The listing builds one solid part. Answer for the finished solid, in the listing's coordinates (mm). Face numbers are marked on the shaded views. Give positions to 0.01 mm unless a question says otherwise; leave off trailing zeros. Loops run counter-clockwise (first coordinate to the right, second up) from the corner with the lowest first, then second, coordinate; pieces in that order, holes last. Notation, with made-up numbers: (62.5, 83.5) - (111.5, 83.5) arc R27 cw to (111.5, 116.5) - close; hole circle Ø10 at (-8.5, 22). An arc over 180 degrees is marked (long way). Answer as CSV lines item,"result". Start each with the question number.
1) A cutting plane is placed at A-A (y = -28.5). Determine the outline of the cut face in (x, z).
2) Find the intervals of material crossed by line 1 along X through (y, z) = (-9.5, 9.25); line 2 along Y through (x, z) = (-28.5, 5.5), in increasing order.
3) For a pull along X with two mould halves and no side action, classify the marked faces 1, 2 and 3 as pulls with the +X half, pulls with the -X half, needs draft (parallel to the pull), parting line crosses it, or undercut.
4) A cutting plane is placed at D-D (y = 22.5). Determine the outline of the cut face in (x, z), and give its area (4 significant figures).
5) A cutting plane is placed at C-C (x = -9). Determine the outline of the cut face in (y, z), and give its area (3 significant figures).
6) A flat-ended cylindrical pin translates along its axis: pin 1 (4 mm diameter, centred on x = -28.5, y = 28.5, fed in from +Z). Find the tip coordinate at first contact, or state that the pin passes through.
```python
from build123d import *

# Parameters (mm, degrees)
F0_W     = 70
F0_H     = 70
F0_R     = 3.5
F1_DEPTH = 10
F2_W     = 50.5
F2_H     = 50.5
F2_W_2   = 34.5
F2_H_2   = 34.5
F3_DEPTH = 5


with BuildPart() as f1:
    # F0 (on Top) → F1 (new body)
    with BuildSketch(Plane.XY):
        Rectangle(F0_W, F0_H)
        with Locations((28.5, -28.5)):
            Circle(F0_R, mode=Mode.SUBTRACT)
        with Locations((-28.5, 28.5)):
            Circle(F0_R, mode=Mode.SUBTRACT)
    extrude(amount=F1_DEPTH)

    # F2 (on face) → F3 (cut)
    with BuildSketch(Plane.XY.offset(10)):
        Rectangle(F2_W, F2_H)
        Rectangle(F2_W_2, F2_H_2, mode=Mode.SUBTRACT)
    extrude(amount=-F3_DEPTH, mode=Mode.SUBTRACT)


solid = f1.part
```
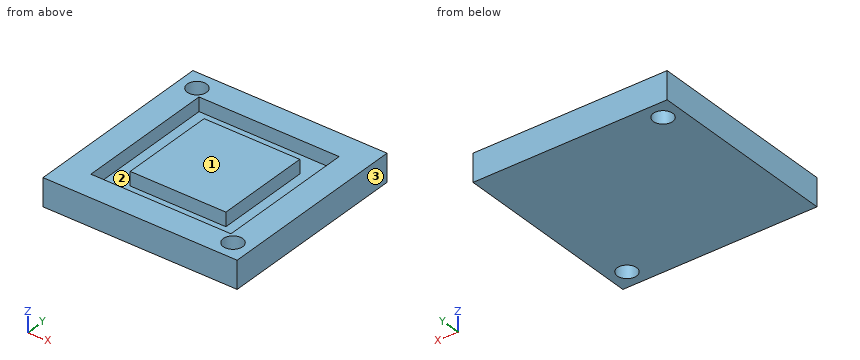
Ans:
1,outline,"(-35, 0) - (25, 0) - (25, 10) - (-35, 10) - close; (32, 0) - (35, 0) - (35, 10) - (32, 10) - close"
2,line 1,"-35 to -25.25, -17.25 to 17.25, 25.25 to 35"
2,line 2,"-35 to 25, 32 to 35"
3,face 1,"needs draft"
3,face 2,"undercut"
3,face 3,"pulls with the +X half"
4,outline,"(-35, 0) - (35, 0) - (35, 10) - (25.25, 10) - (25.25, 5) - (-25.25, 5) - (-25.25, 10) - (-35, 10) - close"
4,area,"447.5 mm2"
5,outline,"(-35, 0) - (35, 0) - (35, 10) - (25.25, 10) - (25.25, 5) - (17.25, 5) - (17.25, 10) - (-17.25, 10) - (-17.25, 5) - (-25.25, 5) - (-25.25, 10) - (-35, 10) - close"
5,area,"620 mm2"
6,pin 1,"through"
